Check sheet for the modelled part. Datum: model origin and axes. Units: mm. A direction names the side the tool comes from. Round coordinates to 2 decimals unless told otherwise and drop trailing zeros. Write each loop counter-clockwise with the first axis right and the second up, starting at its lowest first coordinate (ties: lowest second). Pieces come first, ordered by that corner, then holes. Notation, with made-up numbers: (40, 84.25) -> (80, 84.25) arc R34 cw to (80, 118.25) -> close; hole circle Ø10 at (29, 85.25). An arc over 180 degrees is marked (long way). Put each result on its own line as item: value. Start each with the question number.
from build123d import *

# Parameters (mm, degrees)
SKETCH_2_W          = 17.5
SKETCH_2_H          = 10
EXTRUDE_1_DEPTH     = 125
SKETCH_3_W          = 50
SKETCH_3_H          = 30
EXTRUDE_2_DEPTH     = 7.5
CHAMFER_1_SIZE      = 1
SKETCH_4_R          = 3
CUT_EXTRUDE_1_DEPTH = 10
EXTRUDE_3_DEPTH     = 17.5
CHAMFER_2_SIZE      = 2
CHAMFER_3_SIZE      = 2
SKETCH_6_W          = 10
SKETCH_6_H          = 3
EXTRUDE_4_DEPTH     = 3.1
SKETCH_7_W          = 70
SKETCH_7_H          = 50
EXTRUDE_5_DEPTH     = 3.25
SKETCH_12_W         = 4.5
SKETCH_12_H         = 6
EXTRUDE_6_DEPTH     = 10
CUT_EXTRUDE_4_DEPTH = 10
SKETCH_15_W         = 70
SKETCH_15_H         = 50
CUT_EXTRUDE_7_DEPTH = 0.25
SKETCH_16_W         = 40.5
SKETCH_16_H         = 31.5
CUT_EXTRUDE_8_DEPTH = 39.25
CHAMFER_7_SIZE      = 2
FILLET_1_R          = 1
FILLET_2_R          = 10
EXTRUDE_7_DEPTH     = 3
CUT_EXTRUDE_9_DEPTH = 48


with BuildPart() as part:
    # 草图2 → 凸台-拉伸1 (new body)
    with BuildSketch(Plane(origin=(0, 0, 0), x_dir=(1, 0, 0), z_dir=(0, 1, 0))):
        with Locations((8.75, 5)):
            Rectangle(SKETCH_2_W, SKETCH_2_H)
    extrude(amount=EXTRUDE_1_DEPTH)

    # 草图3 → 凸台-拉伸2 (add)
    with BuildSketch(Plane(origin=(0, 125, 0), x_dir=(1, 0, 0), z_dir=(0, 1, 0))):
        with Locations((8.75, 5)):
            Rectangle(SKETCH_3_W, SKETCH_3_H)
    extrude(amount=EXTRUDE_2_DEPTH)

    # 倒角1
    chamfer_1_edges = [part.edges().sort_by_distance(p)[0] for p in [
        (33.75, 132.5, -5),
        (8.75, 132.5, -20),
        (-16.25, 132.5, -5),
        (8.75, 132.5, 10),
    ]]
    chamfer(chamfer_1_edges, length=CHAMFER_1_SIZE)

    # 草图4 → 切除-拉伸1 (cut)
    with BuildSketch(Plane(origin=(0, 132.5, 0), x_dir=(1, 0, 0), z_dir=(0, 1, 0))):
        with Locations((23.75, 5)):
            Circle(SKETCH_4_R)
        with Locations((-6.25, 5)):
            Circle(SKETCH_4_R)
    extrude(amount=-CUT_EXTRUDE_1_DEPTH, mode=Mode.SUBTRACT)

    # 草图5 → 凸台-拉伸3 (add)
    with BuildSketch(Plane(origin=(17.5, 0, 0), x_dir=(0, 0, -1), z_dir=(1, 0, 0))):
        Polygon((10, 125), (20, 125), (10, 110), align=None)
        Polygon((0, 125), (-10, 125), (0, 110), align=None)
    extrude(amount=-EXTRUDE_3_DEPTH)

    # 倒角2
    chamfer_2_edges = [part.edges().sort_by_distance(p)[0] for p in [
        (-8.125, 125, -20),
        (33.75, 125, -5),
        (-16.25, 125, -5),
        (-8.125, 125, 10),
        (25.625, 125, -20),
        (25.625, 125, 10),
    ]]
    chamfer(chamfer_2_edges, length=CHAMFER_2_SIZE)

    # 倒角3
    chamfer_3_edges = [part.edges().sort_by_distance(p)[0] for p in [
        (0, 55, -10),
        (17.5, 55, -10),
        (17.5, 55, 0),
        (0, 55, 0),
    ]]
    chamfer(chamfer_3_edges, length=CHAMFER_3_SIZE)

    # 草图6 → 凸台-拉伸4 (add)
    with BuildSketch(Plane.XZ):
        with Locations((8.75, -5)):
            Rectangle(SKETCH_6_W, SKETCH_6_H)
    extrude(amount=EXTRUDE_4_DEPTH)

    # 草图7 → 凸台-拉伸5 (add)
    with BuildSketch(Plane.ZY.offset(-8.75)):
        with Locations((-45, 25)):
            Rectangle(SKETCH_7_W, SKETCH_7_H)
    extrude_5 = extrude(amount=EXTRUDE_5_DEPTH)

    # 镜向1: 凸台-拉伸5 across plane
    add(extrude_5.mirror(Plane(origin=(0, 0, -5), x_dir=(1, 0, 0), z_dir=(0, 0, -1))))

    # 草图12 → 凸台-拉伸6 (add)
    with BuildSketch(Plane(origin=(0, 0, -10), x_dir=(-1, 0, 0), z_dir=(0, 0, -1))):
        with Locations((-17.75, 3)):
            Rectangle(SKETCH_12_W, SKETCH_12_H)
    extrude_6 = extrude(amount=-EXTRUDE_6_DEPTH)

    # 镜向2: 凸台-拉伸6 across plane
    add(extrude_6.mirror(Plane.ZY.offset(-8.75)))

    # 草图13 → 切除-拉伸4 (cut)
    with BuildSketch(Plane(origin=(0, 6, 0), x_dir=(1, 0, 0), z_dir=(0, 1, 0))):
        Polygon((17.5, 8), (17.5, 2), (15.5, 0), (20, 0), (20, 10), (15.5, 10), align=None)
    extrude(amount=-CUT_EXTRUDE_4_DEPTH, mode=Mode.SUBTRACT)

    # 草图15 → 切除-拉伸7 (cut)
    with BuildSketch(Plane(origin=(8.75, 0, 0), x_dir=(0, 0, -1), z_dir=(1, 0, 0))):
        with Locations((-35, 25)):
            Rectangle(SKETCH_15_W, SKETCH_15_H)
        with Locations((45, 25)):
            Rectangle(SKETCH_15_W, SKETCH_15_H)
    extrude(amount=-CUT_EXTRUDE_7_DEPTH, mode=Mode.SUBTRACT)

    # 草图16 → 切除-拉伸8 (cut)
    with BuildSketch(Plane.ZY.offset(-5.5)):
        with Locations((-46.25, 26.75)):
            Rectangle(SKETCH_16_W, SKETCH_16_H)
        with Locations((36.25, 26.75)):
            Rectangle(SKETCH_16_W, SKETCH_16_H)
    extrude(amount=-CUT_EXTRUDE_8_DEPTH, mode=Mode.SUBTRACT)

    # 倒角7
    chamfer_7_edges = [part.edges().sort_by_distance(p)[0] for p in [
        (5.5, 25, -10),
        (5.5, 25, 0),
        (8.5, 25, 0),
        (8.5, 25, -10),
    ]]
    chamfer(chamfer_7_edges, length=CHAMFER_7_SIZE)

    # 圆角1
    fillet_1_edges = [part.edges().sort_by_distance(p)[0] for p in [
        (7, 42.5, -26),
        (7, 11, -26),
        (7, 11, -66.5),
        (7, 42.5, -66.5),
        (7, 11, 16),
        (7, 42.5, 16),
        (7, 42.5, 56.5),
        (7, 11, 56.5),
    ]]
    fillet(fillet_1_edges, radius=FILLET_1_R)

    # 圆角2
    fillet_2_edges = [part.edges().sort_by_distance(p)[0] for p in [
        (7, 50, -80),
        (7, 50, 70),
    ]]
    fillet(fillet_2_edges, radius=FILLET_2_R)

    # 草图17 → 凸台-拉伸7 (add)
    with BuildSketch(Plane(origin=(0, 50, 0), x_dir=(1, 0, 0), z_dir=(0, 1, 0))):
        Polygon((5.5, 70), (-9.5, 20), (-9.5, -10), (5.5, -60), align=None)
    extrude(amount=-EXTRUDE_7_DEPTH)

    # 草图18 → 切除-拉伸9 (cut)
    with BuildSketch(Plane.ZY.offset(-5.5)):
        with BuildLine():
            Line((62.05, 39.5), (62.05, 13))
            ThreePointArc((62.05, 13), (59.9, 10.85), (57.75, 13))
            Line((57.75, 13), (57.75, 39.5))
            ThreePointArc((57.75, 39.5), (59.9, 41.65), (62.05, 39.5))
        make_face()
        with BuildLine():
            Line((10.45, 39.5), (10.45, 13))
            ThreePointArc((10.45, 13), (12.6, 10.85), (14.75, 13))
            Line((14.75, 13), (14.75, 39.5))
            ThreePointArc((14.75, 39.5), (12.6, 41.65), (10.45, 39.5))
        make_face()
        with BuildLine():
            Line((-20.45, 39.5), (-20.45, 13))
            ThreePointArc((-20.45, 13), (-22.6, 10.85), (-24.75, 13))
            Line((-24.75, 13), (-24.75, 39.5))
            ThreePointArc((-24.75, 39.5), (-22.6, 41.65), (-20.45, 39.5))
        make_face()
        with BuildLine():
            Line((-72.05, 39.5), (-72.05, 13))
            ThreePointArc((-72.05, 13), (-69.9, 10.85), (-67.75, 13))
            Line((-67.75, 13), (-67.75, 39.5))
            ThreePointArc((-67.75, 39.5), (-69.9, 41.65), (-72.05, 39.5))
        make_face()
    extrude(amount=-CUT_EXTRUDE_9_DEPTH, mode=Mode.SUBTRACT)


solid = part.part
1. Gauge pin test, flat ends, axial feed: P1, Ø1, axis at y = 35.5, z = -15, coming from the -X side; P2, Ø4, axis at x = 4.5, z = -32.5, coming from the -Y side; P3, Ø10, axis at y = 50.5, z = -16, coming from the -X side; P4, Ø3.5, axis at x = 23.75, z = -5, coming from the -Y side. Record the tip position at first contact, or that the pin passes through.
2. Material ranges on L1, parallel to X at y = 127.75, z = -5; L2, parallel to Z at x = -6, y = 131, recorded low to high. Write a range as [from, to].
3. Section check D-D, the plane x = -6.25. Enter the section's corners in (y, z), then the cut area to 3 significant figures.
4. Draft check along Y on faces 5 (the flat face through (0, 27, -5)), 6 (the flat face through (10, 68, -10)), 7 (the flat face through (5.5, 9, -46)). Enter one of: released by +Y, released by -Y, zero draft, split by the parting line, or undercut.
5. Section check B-B, the plane x = 23.75. Enter the section's corners in (y, z), then the cut area to 3 significant figures.
6. Access from +Z, -Z, +X, -X, +Y, -Y to the whole of each face (thin tool, end or side, straight path). Record for faces 1 (the flat face through (5.5, 9, 36)), 2 (the flat face through (2.3, 18.4, -10)), 3 (the flat face through (8.5, 9, 36)), 4 (the cylindrical face through (-4.866, 128.803, -2.338)).
7. Section check A-A, the plane z = -61. Enter the section's corners in (x, y), then the cut area to 3 significant figures.
8. Section check C-C, the plane y = 94. Enter the section's corners in (x, z), then the cut area to 3 significant figures.
Reply:
1. P1: stops at x = 5.5
1. P2: stops at y = 0
1. P3: stops at x = -9.5
1. P4: passes through
2. L1: x = [-16.25, -9.25], [-3.25, 20.75], [26.75, 33.75]
2. L2: z = [-20, -7.99], [-2.01, 10]
3. outline: (47, -30.83) -> (50, -30.83) -> (50, 20.83) -> (47, 20.83) -> close; (125, -18) -> (127, -20) -> (131.5, -20) -> (132.5, -19) -> (132.5, -8) -> (125, -8) -> close; (125, -2) -> (132.5, -2) -> (132.5, 9) -> (131.5, 10) -> (127, 10) -> (125, 8) -> close
3. area: 330 mm2
4. face 5: undercut
4. face 6: undercut
4. face 7: zero draft
5. outline: (125, -18) -> (127, -20) -> (131.5, -20) -> (132.5, -19) -> (132.5, -8) -> (125, -8) -> close; (125, -2) -> (132.5, -2) -> (132.5, 9) -> (131.5, 10) -> (127, 10) -> (125, 8) -> close
5. area: 175 mm2
6. face 1: +Z, -X, -Y
6. face 2: -Z, -X, -Y
6. face 3: +Z, +X, -Y
6. face 4: +Y
7. outline: (2.8, 47) -> (5.5, 47) -> (5.5, 42.5) -> (8.5, 42.5) -> (8.5, 50) -> (2.8, 50) -> close; (5.5, 0) -> (8.5, 0) -> (8.5, 11) -> (5.5, 11) -> close
7. area: 63.6 mm2
8. outline: (0, -8) -> (2, -10) -> (15.5, -10) -> (17.5, -8) -> (17.5, -2) -> (15.5, 0) -> (2, 0) -> (0, -2) -> close
8. area: 167 mm2
